Part print with two shaded views. Sizes in mm from the minimum x, y, z corner. Round coordinates to 2 decimals unless told otherwise and drop trailing zeros. Loops run counter-clockwise (first coordinate to the right, second up) from the corner with the lowest first, then second, coordinate; pieces in that order, holes last.
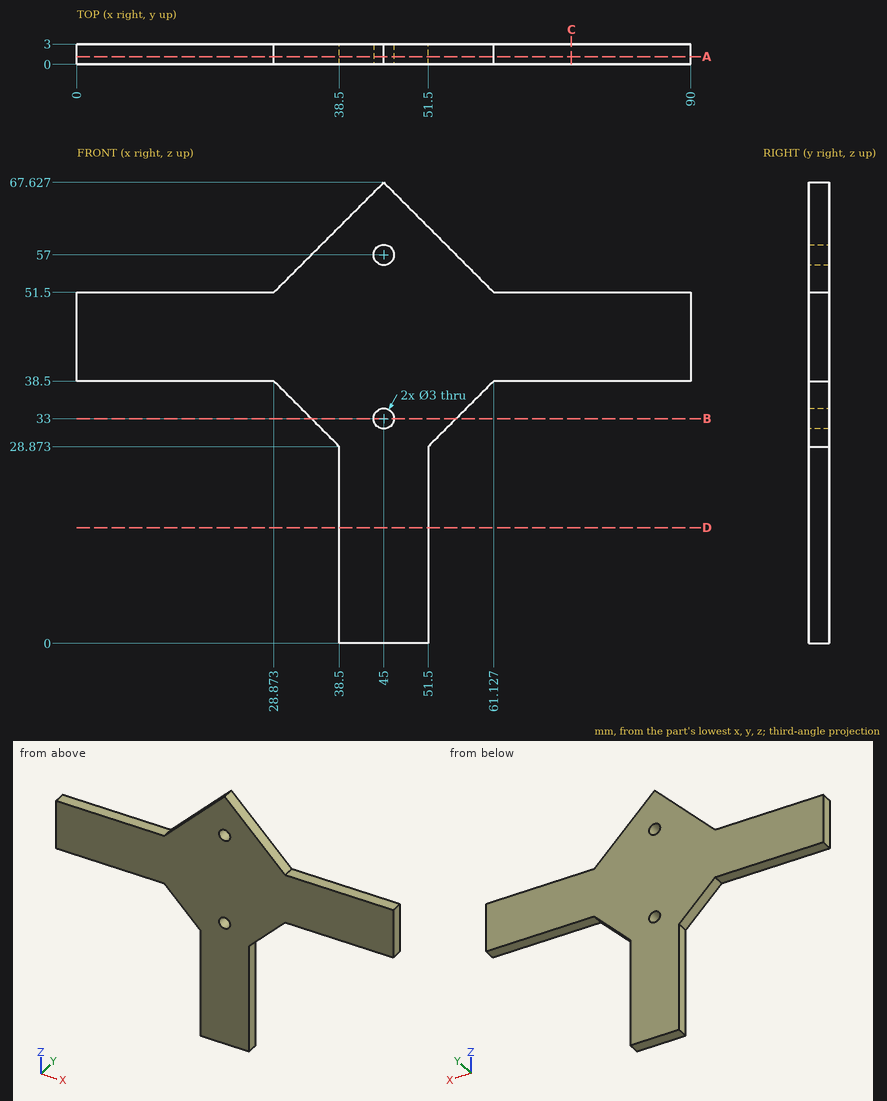
Item 1: Cut at B-B (z = 33). List the corners of the cut face in (x, y).
Verdict:
outline: (34.37, 0) - (43.5, 0) - (43.5, 3) - (34.37, 3) - close; (46.5, 0) - (55.63, 0) - (55.63, 3) - (46.5, 3) - close
Item 2: Wall check: L1, parallel to X at y = 0.8, z = 12; L2, parallel to X at y = 2.65, z = 33.5 (1 decimal). Give the ranges that are in metal, low to high.
Verdict:
L1: x = 38.5 to 51.5
L2: x = 33.9 to 43.6, 46.4 to 56.1
Item 3: Cut at A-A (y = 1.15). List the corners of the cut face in (x, z), plus the area to 3 significant figures.
Verdict:
outline: (0, 38.5) - (28.87, 38.5) - (38.5, 28.87) - (38.5, 0) - (51.5, 0) - (51.5, 28.87) - (61.13, 38.5) - (90, 38.5) - (90, 51.5) - (61.13, 51.5) - (45, 67.63) - (28.87, 51.5) - (0, 51.5) - close; hole circle Ø3 at (45, 33); hole circle Ø3 at (45, 57)
area: 2,010 mm2
Item 4: Cut at C-C (x = 72.5). List the corners of the cut face in (y, z).
Verdict:
outline: (0, 38.5) - (3, 38.5) - (3, 51.5) - (0, 51.5) - close
Item 5: Cut at D-D (z = 17). List the corners of the cut face in (x, y), plus the area to 3 significant figures.
Verdict:
outline: (38.5, 0) - (51.5, 0) - (51.5, 3) - (38.5, 3) - close
area: 39.0 mm2
Item 6: Flat gauge pins, fed straight in: P1, Ø1.5, axis at x = 21, y = 1.5, coming from the +Z side; P2, Ø1.5, axis at x = 72.5, y = 2, coming from the -Z side; P3, Ø0.9, axis at y = 1, z = 9.5, coming from the -X side. Where does each tip first touch, or does it go through?
Verdict:
P1: stops at z = 51.5
P2: stops at z = 38.5
P3: stops at x = 38.5
